Part model, mm, in its own coordinate system. A direction names the side the tool comes from. Give positions to 0.01 mm unless a question says otherwise; leave off trailing zeros. Order: outer loops, then holes, each group sorted by start corner. A loop starts at its lowest first (then second) coordinate and runs counter-clockwise, first axis right, second up. Notation, with made-up numbers: (16.25, -6.5) -> (48.25, -6.5) arc R35 ccw to (48.25, 26.5) -> close; hole circle Ø8 at (-33.5, 72). An arc over 180 degrees is marked (long way). Write item = value, one per line. Start each with the question number.
(1) Saw through at A-A, the plane y = 0. List the corners of the cut face in (x, z) (3 decimals).
(2) Flat gauge pins, fed straight in: pin 1 (6 mm diameter, centred on x = -7.5, y = 16.5, fed in from -Z); pin 2 (12 mm diameter, centred on x = 20, y = 21, fed in from +Z) (3 decimals); pin 3 (1.6 mm diameter, centred on x = 17, z = 1.5, fed in from -Y); pin 4 (1 mm diameter, centred on y = 3, z = 2.5, fed in from +X). Where does each tip first touch, or does it go through?
(3) Saw through at D-D, the plane y = -10. List the corners of the cut face in (x, z) (3 decimals), then the cut area to 3 significant figures.
(4) Saw through at B-B, the plane z = 2.1. List the corners of the cut face in (x, y) (3 decimals), then the cut area to 3 significant figures.
(5) Which spindle directions (+Z, -Z, +X, -X, +Y, -Y) get a long thin tool onto all of the face, cutting with end or side? Do faces 1 (the cylindrical face through (-5.716, 5.778, 1.565)), 2 (the flat face through (0, -7, 0)). Say none if no direction does.
(6) Two-plate mould, pull along X, no slides. Class faces 3 (the flat face through (0, -7, 3.175)), 4 (the flat face through (3.175, 18, 2)), 5 (the cylindrical face through (31.5, 9.9, 1.6)): pulls with the +X half, pulls with the -X half, needs draft (parallel to the pull), parting line crosses it, or undercut.
(7) Probe line 1 along Y through (x, z) = (0, 1.9); line 2 along X through (y, z) = (-13, 2.3) (3 decimals); line 3 along Y through (x, z) = (11.5, 1.7) (3 decimals). List the from-to ranges inside material, lowest first. Write a range as from..to.
from build123d import *

# Parameters (mm, degrees)
SKETCH1_R           = 33.02
SKETCH1_R_2         = 4.953
BOSS_EXTRUDE1_DEPTH = 3.175


with BuildPart() as part:
    # Sketch1 → Boss-Extrude1 (new body)
    with BuildSketch(Plane.XY):
        Circle(SKETCH1_R)
        Circle(SKETCH1_R_2, mode=Mode.SUBTRACT)
        with BuildLine():
            Line((-7.482229547, 3.175), (-29.675636472, 3.175))
            ThreePointArc((-29.675636472, 3.175), (-21.103601885, 21.103601885), (-3.175, 29.675636472))
            Line((-3.175, 29.675636472), (-3.175, 7.482229547))
            ThreePointArc((-3.175, 7.482229547), (-5.747363917, 5.747363917), (-7.482229547, 3.175))
        make_face(mode=Mode.SUBTRACT)
        with BuildLine():
            Line((3.175, 7.482229547), (3.175, 29.675636472))
            ThreePointArc((3.175, 29.675636472), (21.103601885, 21.103601885), (29.675636472, 3.175))
            Line((29.675636472, 3.175), (7.482229547, 3.175))
            ThreePointArc((7.482229547, 3.175), (5.747363917, 5.747363917), (3.175, 7.482229547))
        make_face(mode=Mode.SUBTRACT)
        with BuildLine():
            Line((7.482229547, -3.175), (29.675636472, -3.175))
            ThreePointArc((29.675636472, -3.175), (21.103601885, -21.103601885), (3.175, -29.675636472))
            Line((3.175, -29.675636472), (3.175, -7.482229547))
            ThreePointArc((3.175, -7.482229547), (5.747363917, -5.747363917), (7.482229547, -3.175))
        make_face(mode=Mode.SUBTRACT)
        with BuildLine():
            Line((-3.175, -7.482229547), (-3.175, -29.675636472))
            ThreePointArc((-3.175, -29.675636472), (-21.103601885, -21.103601885), (-29.675636472, -3.175))
            Line((-29.675636472, -3.175), (-7.482229547, -3.175))
            ThreePointArc((-7.482229547, -3.175), (-5.747363917, -5.747363917), (-3.175, -7.482229547))
        make_face(mode=Mode.SUBTRACT)
    extrude(amount=BOSS_EXTRUDE1_DEPTH)


solid = part.part
Results list:
q1.outline = (-33.02, 0) -> (-4.953, 0) -> (-4.953, 3.175) -> (-33.02, 3.175) -> close; (4.953, 0) -> (33.02, 0) -> (33.02, 3.175) -> (4.953, 3.175) -> close
q2.pin_1 = through
q2.pin_2 = 3.175
q2.pin_3 = -28.77
q2.pin_4 = 32.93
q3.outline = (-31.469, 0) -> (-28.12, 0) -> (-28.12, 3.175) -> (-31.469, 3.175) -> close; (-3.175, 0) -> (3.175, 0) -> (3.175, 3.175) -> (-3.175, 3.175) -> close; (28.12, 0) -> (31.469, 0) -> (31.469, 3.175) -> (28.12, 3.175) -> close
q3.area = 41.4 mm^2
q4.outline = circle Ø66.04 at (0, 0); hole (-29.676, -3.175) arc R29.845 ccw to (-3.175, -29.676) -> (-3.175, -7.482) arc R8.128 cw to (-7.482, -3.175) -> close; hole (-29.676, 3.175) -> (-7.482, 3.175) arc R8.128 cw to (-3.175, 7.482) -> (-3.175, 29.676) arc R29.845 ccw to start; hole circle Ø9.906 at (0, 0); hole (3.175, -29.676) arc R29.845 ccw to (29.676, -3.175) -> (7.482, -3.175) arc R8.128 cw to (3.175, -7.482) -> close; hole (3.175, 7.482) arc R8.128 cw to (7.482, 3.175) -> (29.676, 3.175) arc R29.845 ccw to (3.175, 29.676) -> close
q4.area = 1,310 mm^2
q5.face_1 = +Z, -Z
q5.face_2 = -Z, +X, -X, +Y, -Y
q6.face_3 = needs draft
q6.face_4 = undercut
q6.face_5 = parting line crosses it
q7.line_1 = -33.02..-4.95, 4.95..33.02
q7.line_2 = -30.353..-26.865, -3.175..3.175, 26.865..30.353
q7.line_3 = -30.953..-27.54, -3.175..3.175, 27.54..30.953
